Geometry check sheet. Reference: the model listing, model coordinates, mm. A direction names the side the tool comes from. Coordinates: 2 decimals unless noted, no trailing zeros. Write each loop counter-clockwise with the first axis right and the second up, starting at its lowest first coordinate (ties: lowest second). Pieces come first, ordered by that corner, then holes.
Autodesk Fusion 360 part; units mm, degrees
sketch "Sketch1" plane through (0, 0, 0) normal (0, 1, 0) x (1, 0, 0) in component "Circle Out"
  circle A0 centre (0, 0) radius 50
  circle A1 centre (0, 0) radius 40
  circle A2 centre (0, 0) radius 4.5
  line L0 (11.5858, -14.4142) -> (2, -4.8284)
  line L1 (2, -20) -> (2, -39.95)
  line L2 (11.5858, -14.4142) -> (26.8347, -29.6631)
  line L3 (-2, -20) -> (-2, -39.95)
  line L4 (14.4142, -11.5858) -> (29.6631, -26.8347)
  line L5 (24, -2) -> (4.8284, -2)
  line L6 (24, -2) -> (39.95, -2)
  line L7 (24, 2) -> (39.95, 2)
  line L8 (16.7362, 13.9078) -> (4.8284, 2)
  line L9 (16.7362, 13.9078) -> (29.6631, 26.8347)
  line L10 (13.9078, 16.7362) -> (26.8347, 29.6631)
  line L11 (2, 15) -> (2, 4.8284)
  line L12 (2, 15) -> (2, 39.95)
  line L13 (-2, 15) -> (-2, 39.95)
  line L14 (-8.5858, 11.4142) -> (-2, 4.8284)
  line L15 (-8.5858, 11.4142) -> (-26.8347, 29.6631)
  line L16 (-11.4142, 8.5858) -> (-11.591, 8.7626)
  line L17 (-11.591, 8.7626) -> (-29.6631, 26.8347)
  line L18 (-14, 2) -> (-4.8284, 2)
  line L19 (-14, 2) -> (-39.95, 2)
  line L20 (-14, -2) -> (-39.95, -2)
  line L21 (-13.0052, -10.1768) -> (-4.8284, -2)
  line L22 (-13.0052, -10.1768) -> (-29.6631, -26.8347)
  line L23 (-10.1768, -13.0052) -> (-26.8347, -29.6631)
  line L24 (-10.1768, -13.0052) -> (-2, -4.8284)
  line L25 (-2, -4.8284) -> (-2, -39.95)
  line L26 (2, -4.8284) -> (2, -20)
  line L27 (4.8284, -2) -> (14.4142, -11.5858)
  line L28 (4.8284, 2) -> (24, 2)
  line L29 (2, 4.8284) -> (13.9078, 16.7362)
  line L30 (-2, 4.8284) -> (-2, 15)
  line L31 (-4.8284, 2) -> (-11.4142, 8.5858)
  line L32 (-14, -2) -> (-4.8284, -2)
  dimension "d2" = 100
  dimension "d3" = 9
extrude "Extrude1" add sketch "Sketch1" along normal blind 5 contours A0 | A1 L0 L1 L2 L3 L4 L5 L6 L7 L8 L9 L10 L11 L12 L13 L14 L15 L16 L17 L18 L19 L20 L21 L22 L23 L24 L25 L26 L27 L28 L29 L30 L31 L32 | A2 in component "Circle Out"
sketch "Sketch2" plane through (0, 5, 0) normal (0, 1, 0) x (-1, 0, 0) in component "Circle Out"
  line L0 (4.8284, -2) -> (39.95, -2)
  arc A0 (29.6631, -26.8347) -> (39.95, -2) centre (0, 0) ccw
  line L1 (29.6631, -26.8347) -> (4.8284, -2)
  line L2 (-2, -4.8284) -> (-2, -39.95)
  arc A1 (-26.8347, -29.6631) -> (-2, -39.95) centre (0, 0) ccw
  line L3 (-26.8347, -29.6631) -> (-2, -4.8284)
  line L4 (2, -4.8284) -> (26.8347, -29.6631)
  arc A2 (2, -39.95) -> (26.8347, -29.6631) centre (0, 0) ccw
  line L5 (2, -39.95) -> (2, -4.8284)
  line L6 (-4.8284, -2) -> (-29.6631, -26.8347)
  arc A3 (-39.95, -2) -> (-29.6631, -26.8347) centre (0, 0) ccw
  line L7 (-39.95, -2) -> (-4.8284, -2)
  arc A4 (39.95, 2) -> (29.6631, 26.8347) centre (0, 0) ccw
  line L8 (39.95, 2) -> (4.8284, 2)
  line L9 (4.8284, 2) -> (29.6631, 26.8347)
  line L10 (-4.8284, 2) -> (-39.95, 2)
  arc A5 (-29.6631, 26.8347) -> (-39.95, 2) centre (0, 0) ccw
  line L11 (-29.6631, 26.8347) -> (-4.8284, 2)
  line L12 (26.8347, 29.6631) -> (2, 4.8284)
  line L13 (2, 4.8284) -> (2, 39.95)
  arc A6 (26.8347, 29.6631) -> (2, 39.95) centre (0, 0) ccw
  line L14 (-2, 4.8284) -> (-26.8347, 29.6631)
  arc A7 (-2, 39.95) -> (-26.8347, 29.6631) centre (0, 0) ccw
  line L15 (-2, 39.95) -> (-2, 4.8284)
  circle A8 centre (0, 0) radius 50
  circle A9 centre (0, 0) radius 4.25
  dimension "d25" = 8.5
extrude "Extrude2" add sketch "Sketch2" along normal blind 9 contours A9 in component "Circle Out"
sketch "Sketch3" plane through (0, 14, 0) normal (0, 1, 0) x (-1, 0, 0) in component "Circle Out"
  circle A0 centre (0, 0) radius 4.25
  line L0 (-2, 0) -> (-2, 1.3)
  line L1 (-2, 1.3) -> (0, 2)
  line L2 (2, 0) -> (2, 1.3)
  line L3 (2, 1.3) -> (0, 2)
  line L4 (-2, 0) -> (-2, -1.3)
  line L5 (-2, -1.3) -> (0, -2)
  line L6 (2, 0) -> (2, -1.3)
  line L7 (2, -1.3) -> (0, -2)
extrude "Extrude3" cut sketch "Sketch3" against normal blind 16 contours L0 L1 L2 L3 L4 L5 L6 L7 in component "Circle Out"
sketch "Sketch4" plane through (0, 0, 0) normal (0, -1, 0) x (1, 0, 0) in component "Circle Out"
  line L0 (-2, 1.3) -> (0, 2)
  line L1 (0, 2) -> (2, 1.3)
  line L2 (2, 1.3) -> (2, -1.3)
  line L3 (2, -1.3) -> (0, -2)
  line L4 (0, -2) -> (-2, -1.3)
  line L5 (-2, -1.3) -> (-2, 1.3)
  line L6 (-39.95, -2) -> (-4.8284, -2)
  line L7 (-4.8284, -2) -> (-29.6631, -26.8347)
  arc A0 (-39.95, -2) -> (-29.6631, -26.8347) centre (0, 0) ccw
  line L8 (2, -39.95) -> (2, -4.8284)
  line L9 (2, -4.8284) -> (26.8347, -29.6631)
  arc A1 (2, -39.95) -> (26.8347, -29.6631) centre (0, 0) ccw
  line L10 (-26.8347, -29.6631) -> (-2, -4.8284)
  line L11 (-2, -4.8284) -> (-2, -39.95)
  arc A2 (-26.8347, -29.6631) -> (-2, -39.95) centre (0, 0) ccw
  line L12 (29.6631, -26.8347) -> (4.8284, -2)
  line L13 (4.8284, -2) -> (39.95, -2)
  arc A3 (29.6631, -26.8347) -> (39.95, -2) centre (0, 0) ccw
  arc A4 (-29.6631, 26.8347) -> (-39.95, 2) centre (0, 0) ccw
  line L14 (-29.6631, 26.8347) -> (-4.8284, 2)
  line L15 (-4.8284, 2) -> (-39.95, 2)
  line L16 (39.95, 2) -> (4.8284, 2)
  line L17 (4.8284, 2) -> (29.6631, 26.8347)
  arc A5 (39.95, 2) -> (29.6631, 26.8347) centre (0, 0) ccw
  line L18 (-2, 4.8284) -> (-26.8347, 29.6631)
  arc A6 (-2, 39.95) -> (-26.8347, 29.6631) centre (0, 0) ccw
  line L19 (-2, 39.95) -> (-2, 4.8284)
  line L20 (26.8347, 29.6631) -> (2, 4.8284)
  line L21 (2, 4.8284) -> (2, 39.95)
  arc A7 (26.8347, 29.6631) -> (2, 39.95) centre (0, 0) ccw
  circle A8 centre (0, 0) radius 50
  circle A9 centre (-17.2208, 41.5746) radius 2.5
  circle A10 centre (-41.5746, 17.2208) radius 2.5
  circle A11 centre (-41.5746, -17.2208) radius 2.5
  circle A12 centre (-17.2208, -41.5746) radius 2.5
  circle A13 centre (17.2208, -41.5746) radius 2.5
  circle A14 centre (41.5746, -17.2208) radius 2.5
  circle A15 centre (41.5746, 17.2208) radius 2.5
  circle A16 centre (17.2208, 41.5746) radius 2.5
  dimension "d32" = 5
  dimension "d33" = 5
  dimension "d34" = 5
  dimension "d35" = 5
  dimension "d36" = 5
  dimension "d37" = 5
  dimension "d38" = 5
  dimension "d39" = 5
extrude "Extrude4" cut sketch "Sketch4" against normal blind 10 contours A9 | A10 | A11 | A12 | A13 | A14 | A15 | A16 in component "Circle Out"
sketch "Sketch5" plane through (0, 5, 0) normal (0, 1, 0) x (-1, 0, 0) in component "Circle Out"
  circle A0 centre (-41.5746, 17.2208) radius 2.5
  circle A1 centre (41.5746, -17.2208) radius 2.5
  circle A2 centre (17.2208, -41.5746) radius 2.5
  circle A3 centre (-17.2208, 41.5746) radius 2.5
  circle A4 centre (-41.5746, -17.2208) radius 2.5
  circle A5 centre (41.5746, 17.2208) radius 2.5
  circle A6 centre (-17.2208, -41.5746) radius 2.5
  circle A7 centre (17.2208, 41.5746) radius 2.5
  circle A8 centre (0, 0) radius 4.25
  line L0 (4.8284, -2) -> (39.95, -2)
  arc A9 (29.6631, -26.8347) -> (39.95, -2) centre (0, 0) ccw
  line L1 (29.6631, -26.8347) -> (4.8284, -2)
  line L2 (-2, -4.8284) -> (-2, -39.95)
  arc A10 (-26.8347, -29.6631) -> (-2, -39.95) centre (0, 0) ccw
  line L3 (-26.8347, -29.6631) -> (-2, -4.8284)
  line L4 (2, -4.8284) -> (26.8347, -29.6631)
  arc A11 (2, -39.95) -> (26.8347, -29.6631) centre (0, 0) ccw
  line L5 (2, -39.95) -> (2, -4.8284)
  line L6 (-4.8284, -2) -> (-29.6631, -26.8347)
  arc A12 (-39.95, -2) -> (-29.6631, -26.8347) centre (0, 0) ccw
  line L7 (-39.95, -2) -> (-4.8284, -2)
  arc A13 (39.95, 2) -> (29.6631, 26.8347) centre (0, 0) ccw
  line L8 (39.95, 2) -> (4.8284, 2)
  line L9 (4.8284, 2) -> (29.6631, 26.8347)
  line L10 (-4.8284, 2) -> (-39.95, 2)
  arc A14 (-29.6631, 26.8347) -> (-39.95, 2) centre (0, 0) ccw
  line L11 (-29.6631, 26.8347) -> (-4.8284, 2)
  line L12 (26.8347, 29.6631) -> (2, 4.8284)
  line L13 (2, 4.8284) -> (2, 39.95)
  arc A15 (26.8347, 29.6631) -> (2, 39.95) centre (0, 0) ccw
  line L14 (-2, 4.8284) -> (-26.8347, 29.6631)
  arc A16 (-2, 39.95) -> (-26.8347, 29.6631) centre (0, 0) ccw
  line L15 (-2, 39.95) -> (-2, 4.8284)
  circle A17 centre (0, 0) radius 50
  circle A18 centre (-17.2208, 41.5746) radius 4.25
  circle A19 centre (17.2208, 41.5746) radius 4.25
  circle A20 centre (-41.5746, 17.2208) radius 4.25
  circle A21 centre (-41.5746, -17.2208) radius 4.25
  circle A22 centre (-17.2208, -41.5746) radius 4.25
  circle A23 centre (17.2208, -41.5746) radius 4.25
  circle A24 centre (41.5746, -17.2208) radius 4.25
  circle A25 centre (41.5746, 17.2208) radius 4.25
  dimension "d42" = 8.5
  dimension "d43" = 8.5
  dimension "d44" = 8.5
  dimension "d45" = 8.5
  dimension "d46" = 8.5
  dimension "d47" = 8.5
  dimension "d48" = 8.5
  dimension "d49" = 8.5
extrude "Extrude5" cut sketch "Sketch5" against normal blind 2.5 contours A18 | A19 | A20 | A21 | A22 | A23 | A24 | A25 in component "Circle Out"
component "Circle Out" placed x (1, 0, 0) y (0, 1, 0) z (0, 0, 1) at (0, 0, 0)
1. Sectioned sample at B-B, the plane z = 0. Record the boundary of the cut face in (x, y).
Computed values:
outline: (-50, 0) - (-2, 0) - (-2, 14) - (-4.25, 14) - (-4.25, 5) - (-50, 5) - close; (2, 0) - (50, 0) - (50, 5) - (4.25, 5) - (4.25, 14) - (2, 14) - close
2. Draft check along X on faces 3 (the flat face through (17.07, 2.46, -14.24)), 4 (the cylindrical face through (-2.285, 9.437, -3.584)). Enter one of: released by +X, released by -X, zero draft, split by the parting line, or undercut.
Computed values:
face 3: undercut
face 4: split by the parting line
3. Sectioned sample at D-D, the plane x = -42.5. Record the boundary of the cut face in (y, z), and give its area (3 significant figures).
Computed values:
outline: (0, -26.34) - (5, -26.34) - (5, -21.37) - (2.5, -21.37) - (2.5, -19.54) - (0, -19.54) - close; (0, -14.9) - (2.5, -14.9) - (2.5, -13.07) - (5, -13.07) - (5, 13.07) - (2.5, 13.07) - (2.5, 14.9) - (0, 14.9) - close; (0, 19.54) - (2.5, 19.54) - (2.5, 21.37) - (5, 21.37) - (5, 26.34) - (0, 26.34) - close
area: 199 mm2
4. Thickness scan on line 1 along X through (y, z) = (1.5, 43.5); line 2 along Y through (x, z) = (15, 46.5); line 3 along Z through (x, y) = (28, 3.75). Record the ranges inside material, lowest first.
Computed values:
line 1: x = -24.65 to -18.82, -15.63 to 15.63, 18.82 to 24.65
line 2: y = 0 to 5
line 3: z = -41.42 to -25.17, -2 to 2, 25.17 to 41.42
5. Sectioned sample at A-A, the plane y = 8.5. Record the boundary of the cut face in (x, z), and give its area (3 significant figures).
Computed values:
outline: circle Ø8.5 at (0, 0); hole (-2, -1.3) - (0, -2) - (2, -1.3) - (2, 1.3) - (0, 2) - (-2, 1.3) - close
area: 43.5 mm2
6. Access from +Z, -Z, +X, -X, +Y, -Y to the whole of each face (thin tool, end or side, straight path). Record for faces 1 (the flat face through (-2, 7, 0)), 2 (the cylindrical face through (18.142, 3.768, -45.724)).
Computed values:
face 1: +Y, -Y
face 2: +Y
7. Sectioned sample at C-C, the plane x = 23. Record the boundary of the cut face in (y, z).
Computed values:
outline: (0, -44.4) - (5, -44.4) - (5, -32.73) - (0, -32.73) - close; (0, -25.83) - (5, -25.83) - (5, -20.17) - (0, -20.17) - close; (0, -2) - (5, -2) - (5, 2) - (0, 2) - close; (0, 20.17) - (5, 20.17) - (5, 25.83) - (0, 25.83) - close; (0, 32.73) - (5, 32.73) - (5, 44.4) - (0, 44.4) - close
8. Gauge pin test, flat ends, axial feed: pin 1 Ø1.5 at (y, z) = (3, 16) entering from -X; pin 2 Ø10 at (x, z) = (17.22, 41.57) entering from +Y; pin 3 Ø3 at (y, z) = (9.5, 0.5) entering from +X; pin 4 Ø2 at (y, z) = (6.5, -18) entering from +X. Record the tip position at first contact, or that the pin passes through.
Computed values:
pin 1: stops at x = -47.62
pin 2: stops at y = 5
pin 3: stops at x = 4.25
pin 4: passes through
